CAD build for the part. Positions are in the model's coordinates, mm. A direction names the side the tool comes from. Give positions to 0.01 mm unless a question says otherwise; leave off trailing zeros. Loops run counter-clockwise (first coordinate to the right, second up) from the corner with the lowest first, then second, coordinate; pieces in that order, holes last.
Solid Edge part; units mm, degrees
sketch "Sketch1" plane through (0, 0, 0) normal (0, -1, 0) x (1, 0, 0)
  line L0 (-5, 20) -> (-12, 20)
  line L1 (-12, 20) -> (-12, 27)
  line L2 (-12, 27) -> (-27.75, 27)
  line L3 (-27.75, 27) -> (-27.75, 31)
  line L4 (-27.75, 31) -> (-23.75, 31)
  line L5 (-23.75, 31) -> (-23.75, 29)
  line L6 (-23.75, 29) -> (-19.95, 29)
  line L7 (-19.95, 29) -> (-19.95, 31)
  line L8 (-19.95, 31) -> (-12, 31)
  line L9 (-12, 31) -> (-12, 48)
  line L10 (-12, 48) -> (-1.1, 48)
  line L11 (-1.1, 48) -> (-1.1, 30)
  line L12 (-1.1, 30) -> (0, 30)
  line L13 (0, 30) -> (0, 17.5)
  line L14 (0, 17.5) -> (-5, 17.5)
  line L15 (-5, 17.5) -> (-5, 20)
revolve "RevolvedProtrusion1" add sketch "Sketch1" angle 360 about axis through (0, 0, 0) along (1, 0, 0)
chamfer "Chamfer_1" distance 2 angle 20 1 edges at (-12, 0, -20) measured on face at (-12, 17.46, 18.54)
fillet "Round_1" radius 0.3 4 edges at (-19.95, 0, -31) (-23.75, 0, -31) (-19.95, 0, -29) (-23.75, 0, -29)
chamfer "Chamfer_2" distance 0.5 angle 45 1 edges at (-27.75, 0, -31)
pattern "Pattern1" [suppressed]
hole "Hole_4" at (-1.1, 0, 41) direction (-1, 0, 0) diameter 7 depth 50.8
pattern_circular "Pattern2" count 5 over 360 about axis through (-1.1, 0, 0) along (-1, 0, 0) of "Hole_4"
sketch "Sketch2" plane through (-1.1, 0, 0) normal (1, 0, 0) x (0, 1, 0)
  circle A0 centre (0, 41) radius 5.5
extrude "ExtrudedCutout_1" cut sketch "Sketch2" against normal blind 6.4
pattern_circular "Pattern3" count 5 over 360 about axis through (-1.1, 0, 0) along (-1, 0, 0) of "ExtrudedCutout_1"
1. Pull direction Y, two halves, no side cores. Call faces 5 (the face through (-4.255, 27.884, -37.161)), 6 (the face through (-27.75, 25, 11)), 7 (the face through (-25.628, -30.736, -4.036)): released by +Y, released by -Y, zero draft, split by the parting line, or undercut.
Responses:
face 5: undercut
face 6: zero draft
face 7: split by the parting line
2. Probe line 1 along Z through (x, y) = (-8.85, 0); line 2 along Z through (x, y) = (-3.5, 0); line 3 along Y through (x, z) = (-18, -1). List the from-to ranges inside material, lowest first.
Responses:
line 1: z = -48 to -20, 20 to 37.5, 44.5 to 48
line 2: z = -48 to -17.5, 17.5 to 35.5, 46.5 to 48
line 3: y = -30.98 to -26.98, 26.98 to 30.98
3. Drop flat-ended pins along their axis: pin 1 (8 mm diameter, centred on y = 24.1, z = -33.17, fed in from -X); pin 2 (1.5 mm diameter, centred on y = 30, z = -37, fed in from +X); pin 3 (3 mm diameter, centred on x = -18.5, y = -26.5, fed in from +Z); pin 4 (5.5 mm diameter, centred on y = -24.1, z = -33.17, fed in from -X). Give the stop position or say it passes through.
Responses:
pin 1: stops at x = -12
pin 2: stops at x = -1.1
pin 3: stops at z = 18.33
pin 4: passes through
4. Tool access for faces 1 (the face through (-9.8, -35.5, 12.9)), 2 (the face through (-19.95, 16, 25)), 3 (the face through (-5, 18, 0)), 4 (the face through (-4.26, -44.4, 13.67)): list every direction of +Z, -Z, +X, -X, +Y, -Y with a clear straight run to the whole face (end or side of a thin tool).
Responses:
face 1: +X, -X
face 2: none
face 3: -X
face 4: +X
5. Saw through at A-A, the plane y = 39.5. List the corners of the cut face in (x, z), and give its area (3 significant figures).
Responses:
outline: (-12, -27.27) - (-1.1, -27.27) - (-1.1, 7.19) - (-7.5, 7.19) - (-7.5, 9.21) - (-12, 9.21) - close; (-12, 16.13) - (-7.5, 16.13) - (-7.5, 18.15) - (-1.1, 18.15) - (-1.1, 27.27) - (-12, 27.27) - close
area: 493 mm2
6. Saw through at B-B, the plane x = -16.25. List the corners of the cut face in (y, z).
Responses:
outline: circle Ø62 at (0, 0); hole circle Ø54 at (0, 0)
7. Saw through at D-D, the plane x = -2.25. List the corners of the cut face in (y, z), and give its area (3 significant figures).
Responses:
outline: circle Ø96 at (0, 0); hole circle Ø11 at (-38.99, 12.67); hole circle Ø11 at (-24.1, -33.17); hole circle Ø35 at (0, 0); hole circle Ø11 at (0, 41); hole circle Ø11 at (24.1, -33.17); hole circle Ø11 at (38.99, 12.67)
area: 5,800 mm2
8. Saw through at C-C, the plane z = 41. List the corners of the cut face in (x, y), and give its area (3 significant figures).
Responses:
outline: (-12, -24.96) - (-1.1, -24.96) - (-1.1, -5.5) - (-7.5, -5.5) - (-7.5, -3.5) - (-12, -3.5) - close; (-12, 3.5) - (-7.5, 3.5) - (-7.5, 5.5) - (-1.1, 5.5) - (-1.1, 24.96) - (-12, 24.96) - close
area: 442 mm2
